The model under review builds one solid part; all positions refer to its coordinate system, in mm. A direction names the side the tool comes from. Coordinates: 2 decimals unless noted, no trailing zeros. Write each loop counter-clockwise with the first axis right and the second up, starting at its lowest first coordinate (ties: lowest second). Pieces come first, ordered by that corner, then holes.
```python
from build123d import *

# Parameters (mm, degrees)
BOSS_EXTRUDE1_DEPTH = 1.9
BOSS_EXTRUDE2_DEPTH = 5
SKETCH4_W           = 79.3
SKETCH4_H           = 1.9
BOSS_EXTRUDE3_DEPTH = 1.18
SKETCH5_W           = 79.3
SKETCH5_H           = 1.9
BOSS_EXTRUDE4_DEPTH = 1.18
CHAMFER2_SIZE       = 1.18


with BuildPart() as part:
    # Sketch3 → Boss-Extrude1 (new body)
    with BuildSketch(Plane.XY):
        with BuildLine():
            Line((-37.828427125, -36.25), (-37.828427125, -38.75))
            Line((-37.828427125, -38.75), (41.471572875, -38.75))
            ThreePointArc((41.471572875, -38.75), (43.592893219, -39.628679656), (44.471572875, -41.75))
            Line((44.471572875, -41.75), (44.471572875, -71.66))
            ThreePointArc((44.471572875, -71.66), (43.592893219, -73.781320344), (41.471572875, -74.66))
            Line((41.471572875, -74.66), (-37.828427125, -74.66))
            Line((-37.828427125, -74.66), (-37.828427125, -77.16))
            Line((-37.828427125, -77.16), (-42.5, -72.16))
            Line((-42.5, -72.16), (-42.5, -41.249558803))
            Line((-42.5, -41.249558803), (-37.828427125, -36.25))
        make_face()
    extrude(amount=BOSS_EXTRUDE1_DEPTH)

    # Sketch3_5 → Boss-Extrude2 (add)
    with BuildSketch(Plane.XY):
        Polygon((-42.5, -41.249558803), (-42.5, -72.16), (-37.828427125, -77.16), (-37.828427125, -74.66), (-40.5, -71.800606658), (-40.5, -41.609141031), (-37.828427125, -38.75), (-37.828427125, -36.25), align=None)
    extrude(amount=BOSS_EXTRUDE2_DEPTH)

    # Sketch4 → Boss-Extrude3 (add)
    with BuildSketch(Plane.XZ.offset(74.66)):
        with Locations((1.821572875, 0.95)):
            Rectangle(SKETCH4_W, SKETCH4_H)
    extrude(amount=BOSS_EXTRUDE3_DEPTH)

    # Sketch5 → Boss-Extrude4 (add)
    with BuildSketch(Plane(origin=(0, -38.75, 0), x_dir=(1, 0, 0), z_dir=(0, 1, 0))):
        with Locations((1.821572875, -0.95)):
            Rectangle(SKETCH5_W, SKETCH5_H)
    extrude(amount=BOSS_EXTRUDE4_DEPTH)

    # Chamfer2
    chamfer2_edges = [part.edges().sort_by_distance(p)[0] for p in [
        (1.821572875, -75.84, 1.9),
        (1.821572875, -37.57, 1.9),
    ]]
    chamfer(chamfer2_edges, length=CHAMFER2_SIZE)


solid = part.part
```
Item 1: Take a section at B-B, the plane y = -63.5. Write out the cut boundary in (x, z), plus the area to 3 significant figures.
Solved:
outline: (-42.5, 0) - (44.47, 0) - (44.47, 1.9) - (-40.5, 1.9) - (-40.5, 5) - (-42.5, 5) - close
area: 171 mm2
Item 2: Machinability: for faces 5 (the face through (-40.5, -57, 3)), 6 (the face through (-37.828, -76, 2)), 7 (the face through (-42.5, -57, 2)), which of the approach directions +Z, -Z, +X, -X, +Y, -Y give a long, thin tool a straight path to every point of the face, cutting with its end or side? Answer none if there is none.
Solved:
face 5: +Z, +X
face 6: +Z, +X, -Y
face 7: +Z, -Z, -X, +Y, -Y
Item 3: Take a section at A-A, the plane z = 3.3. Write out the cut boundary in (x, y), plus the area to 3 significant figures.
Solved:
outline: (-42.5, -72.16) - (-37.83, -77.16) - (-37.83, -74.66) - (-40.5, -71.8) - (-40.5, -41.61) - (-37.83, -38.75) - (-37.83, -36.25) - (-42.5, -41.25) - close
area: 79.5 mm2
Item 4: Mouldability with a two-part tool opening along Y and no side actions: class faces 1 (the face through (-37.828, -37, 2)), 2 (the face through (43.569, -39.605, 0.937)), 3 (the face through (43.616, -73.758, 0.937)), 4 (the face through (-39.183, -40.2, 3.428)) as pulls with the +Y half, pulls with the -Y half, needs draft (parallel to the pull), parting line crosses it, or undercut.
Solved:
face 1: needs draft
face 2: pulls with the +Y half
face 3: pulls with the -Y half
face 4: undercut
Item 5: To check wall thickness, follow line 1 along Z through (x, y) = (1.5, -66); line 2 along X through (y, z) = (-50, 2.4); line 3 along Y through (x, z) = (-35, 0.3). State the ranges of each line that lie inside material, in increasing order.
Solved:
line 1: z = 0 to 1.9
line 2: x = -42.5 to -40.5
line 3: y = -75.84 to -37.57
Item 6: Take a section at C-C, the plane x = -1.5. Write out the cut boundary in (y, z), plus the area to 3 significant figures.
Solved:
outline: (-75.84, 0) - (-37.57, 0) - (-37.57, 0.72) - (-38.75, 1.9) - (-74.66, 1.9) - (-75.84, 0.72) - close
area: 71.3 mm2
Item 7: For pin 1 (3 mm diameter, centred on y = -37.5, z = 1.5, fed in from +X); pin 2 (0.6 mm diameter, centred on y = -75, z = 1, fed in from +X); pin 3 (0.8 mm diameter, centred on y = -75.5, z = 3.5, fed in from +X), all flat-tipped, find the tip position at first contact; note any pin that passes through.
Solved:
pin 1: stops at x = 42.67
pin 2: stops at x = 41.47
pin 3: stops at x = -37.83
